Model file for the job. Use its own axes, mm. A direction names the side the tool comes from. Coordinates: 2 decimals unless noted, no trailing zeros. Loops run counter-clockwise (first coordinate to the right, second up) from the corner with the lowest first, then second, coordinate; pieces in that order, holes last. Notation, with made-up numbers: (-26, 46.5) -> (21, 46.5) arc R31 ccw to (21, 74.5) -> close; hole circle Ø2 at (67.25, 45). An arc over 180 degrees is marked (long way). Use one line per item in the form item = value.
```python
from build123d import *

# Parameters (mm, degrees)
SKETCH_1_W          = 200
SKETCH_1_H          = 40
EXTRUDE_1_DEPTH     = 100
SKETCH_1_3_W        = 200
SKETCH_1_3_H        = 40
EXTRUDE_2_DEPTH     = 130
SKETCH_9_R          = 5
CUT_EXTRUDE_4_DEPTH = 35
CUT_EXTRUDE_4_DRAFT = -1
SKETCH_9_3_R        = 5
CUT_EXTRUDE_5_DEPTH = 25
CUT_EXTRUDE_5_DRAFT = -1
SKETCH_9_4_R        = 5
CUT_EXTRUDE_6_DEPTH = 30
CUT_EXTRUDE_6_DRAFT = -1
SKETCH_10_W         = 200
SKETCH_10_H         = 40
EXTRUDE_3_DEPTH     = 160


with BuildPart() as part:
    # Эскиз1 → Бобышка-Вытянуть1 (new body)
    with BuildSketch(Plane.XY):
        with Locations((100, 20)):
            Rectangle(SKETCH_1_W, SKETCH_1_H)
    extrude(amount=EXTRUDE_1_DEPTH)

    # Эскиз1<3> → Бобышка-Вытянуть2 (add)
    with BuildSketch(Plane.XY):
        with Locations((100, 60)):
            Rectangle(SKETCH_1_3_W, SKETCH_1_3_H)
    extrude(amount=EXTRUDE_2_DEPTH)


with BuildPart() as cut_extrude_4_tool:
    # Эскиз9 → Вырез-Вытянуть4 (with draft: the straight prism first)
    with BuildSketch(Plane(origin=(-3.148281851, 38.970132862, 130), x_dir=(1, 0, 0), z_dir=(0, 0, 1))):
        with Locations((42.471240213, 20)):
            Circle(SKETCH_9_R)
    extrude(amount=-CUT_EXTRUDE_4_DEPTH)
    # Вырез-Вытянуть4: the draft: its side faces are tilted about the plane it starts from
    cut_extrude_4_sides = [cut_extrude_4_tool.faces().sort_by_distance(p)[0] for p in [
        (34.322958362, 58.970132862, 112.5),
    ]]
    draft(cut_extrude_4_sides, Plane(origin=(-3.148281851, 38.970132862, 130), x_dir=(1, 0, 0), z_dir=(0, 0, 1)), CUT_EXTRUDE_4_DRAFT)


with BuildPart() as part_1:
    add(part.part)

    # Вырез-Вытянуть4: cut by cut_extrude_4_tool
    add(cut_extrude_4_tool.part, mode=Mode.SUBTRACT)


with BuildPart() as cut_extrude_5_tool:
    # Эскиз9<3> → Вырез-Вытянуть5 (with draft: the straight prism first)
    with BuildSketch(Plane(origin=(-3.148281851, 38.970132862, 130), x_dir=(1, 0, 0), z_dir=(0, 0, 1))):
        with Locations((157.511612736, 20)):
            Circle(SKETCH_9_3_R)
    extrude(amount=-CUT_EXTRUDE_5_DEPTH)
    # Вырез-Вытянуть5: the draft: its side faces are tilted about the plane it starts from
    cut_extrude_5_sides = [cut_extrude_5_tool.faces().sort_by_distance(p)[0] for p in [
        (149.363330884, 58.970132862, 117.5),
    ]]
    draft(cut_extrude_5_sides, Plane(origin=(-3.148281851, 38.970132862, 130), x_dir=(1, 0, 0), z_dir=(0, 0, 1)), CUT_EXTRUDE_5_DRAFT)


with BuildPart() as part_2:
    add(part_1.part)

    # Вырез-Вытянуть5: cut by cut_extrude_5_tool
    add(cut_extrude_5_tool.part, mode=Mode.SUBTRACT)


with BuildPart() as cut_extrude_6_tool:
    # Эскиз9<4> → Вырез-Вытянуть6 (with draft: the straight prism first)
    with BuildSketch(Plane(origin=(-3.148281851, 38.970132862, 130), x_dir=(1, 0, 0), z_dir=(0, 0, 1))):
        with Locations((100, 20)):
            Circle(SKETCH_9_4_R)
    extrude(amount=-CUT_EXTRUDE_6_DEPTH)
    # Вырез-Вытянуть6: the draft: its side faces are tilted about the plane it starts from
    cut_extrude_6_sides = [cut_extrude_6_tool.faces().sort_by_distance(p)[0] for p in [
        (91.851718149, 58.970132862, 115),
    ]]
    draft(cut_extrude_6_sides, Plane(origin=(-3.148281851, 38.970132862, 130), x_dir=(1, 0, 0), z_dir=(0, 0, 1)), CUT_EXTRUDE_6_DRAFT)


with BuildPart() as part_3:
    add(part_2.part)

    # Вырез-Вытянуть6: cut by cut_extrude_6_tool
    add(cut_extrude_6_tool.part, mode=Mode.SUBTRACT)

    # Эскиз10 → Бобышка-Вытянуть3 (add)
    with BuildSketch(Plane(origin=(0, 0, 0), x_dir=(-1, 0, 0), z_dir=(0, 0, -1))):
        with Locations((-100, 100)):
            Rectangle(SKETCH_10_W, SKETCH_10_H)
    extrude(amount=-EXTRUDE_3_DEPTH)


solid = part_3.part
```
Q1. Pin check, flat tips, straight feed: pin 1 Ø2.5 at (x, y) = (39.5, 58.5) entering from +Z; pin 2 Ø10 at (x, y) = (65, 78.5) entering from +Z; pin 3 Ø12 at (x, y) = (71, 25) entering from +Z; pin 4 Ø10 at (x, y) = (98.5, 60.5) entering from +Z. Stop position of each tip, or through.
Result:
pin_1 = 95
pin_2 = 160
pin_3 = 100
pin_4 = 130
Q2. Mould opens along Y. For faces 4 (the face through (39, 59, 95)), 5 (the face through (95.82, 54.34, 115.21)), 6 (the face through (99, 20, 100)), 7 (the face through (99, 40, 115)) say: released by +Y, released by -Y, zero draft, split by the parting line, or undercut.
Result:
face_4 = undercut
face_5 = undercut
face_6 = zero draft
face_7 = released by -Y
Q3. Which spindle directions (+Z, -Z, +X, -X, +Y, -Y) get a long thin tool onto all of the face, cutting with end or side? Do faces 1 (the face through (101, 80, 145)), 2 (the face through (97, 59, 100)), 3 (the face through (101, 100, 160)). Say none if no direction does.
Result:
face_1 = +Z, +X, -X, -Y
face_2 = +Z
face_3 = +Z, +X, -X, +Y, -Y
Q4. Wall check: line 1 along X through (y, z) = (58.5, 127); line 2 along Z through (x, y) = (172, 75); line 3 along Y through (x, z) = (192.5, 103.5). Give the ranges that are in metal, low to high.
Result:
line_1 = 0 to 34.4, 44.25 to 91.93, 101.78 to 149.44, 159.29 to 200
line_2 = 0 to 130
line_3 = 40 to 120
Q5. Band-saw the part on C-C, the plane y = 71.5. Write the cut outline in (x, z), and give its area (3 significant figures).
Result:
outline = (0, 0) -> (200, 0) -> (200, 130) -> (0, 130) -> close
area = 26,000 mm2
Q6. Band-saw the part on A-A, the plane x = 77.5. Write the cut outline in (y, z).
Result:
outline = (0, 0) -> (120, 0) -> (120, 160) -> (80, 160) -> (80, 130) -> (40, 130) -> (40, 100) -> (0, 100) -> close
Q7. Band-saw the part on B-B, the plane z = 117. Write the cut outline in (x, y).
Result:
outline = (0, 40) -> (200, 40) -> (200, 120) -> (0, 120) -> close; hole circle Ø9.55 at (39.32, 58.97); hole circle Ø9.55 at (96.85, 58.97); hole circle Ø9.55 at (154.36, 58.97)
Q8. Band-saw the part on D-D, the plane y = 11.5. Write the cut outline in (x, z).
Result:
outline = (0, 0) -> (200, 0) -> (200, 100) -> (0, 100) -> close
